Autodesk Inventor part; units mm, degrees
ref_plane "YZ Plane" through (0, 0, 0) normal (1, 0, 0) x (0, 1, 0)
ref_plane "XZ Plane" through (0, 0, 0) normal (0, 1, 0) x (-1, 0, 0)
ref_plane "XY Plane" through (0, 0, 0) normal (0, 0, 1) x (1, 0, 0)
sketch "Sketch1" plane through (0, 0, 0) normal (0, 1, 0) x (-1, 0, 0)
  line L0 (0, 0) -> (-12.7, 0)
  line L1 (-12.7, 0) -> (-12.7, -1.5875)
  line L2 (-12.7, -1.5875) -> (0, -1.5875)
  line L3 (0, -1.5875) -> (0, 0)
  line L4 (0, 0) -> (-4.318, 0)
  line L5 (-4.318, 0) -> (-4.318, -12.7)
  line L6 (-4.318, -12.7) -> (0, -12.7)
  line L7 (0, -12.7) -> (0, 0)
  dimension "d0" = 4.318
  dimension "d1" = 12.7
  dimension "d2" = 12.7
  dimension "d33" = 1.5875
extrude "Extrusion1" add sketch "Sketch1" along normal blind 50.8
sketch "Sketch2" plane through (0, 50.8, 0) normal (0, 1, 0) x (1, 0, 0)
  line L0 (12.7, 0) -> (12.7, 1.5875)
  line L1 (12.7, 1.5875) -> (-4.064, 1.5875)
  line L2 (-4.064, 1.5875) -> (-4.064, -8.5725)
  line L3 (-4.064, -8.5725) -> (12.7, -8.5725)
  line L4 (12.7, -8.5725) -> (12.7, 1.5875)
  line L5 (4.318, 12.7) -> (-4.064, 12.7)
  line L6 (-4.064, 12.7) -> (-4.064, -8.5725)
  line L7 (-4.064, -8.5725) -> (4.318, -8.5725)
  line L8 (4.318, -8.5725) -> (4.318, 12.7)
  dimension "d26" = 10.16
  dimension "d28" = 16.764
extrude "Extrusion2" add sketch "Sketch2" along normal blind 6.35
sketch "Sketch5" plane through (0, 50.8, 0) normal (0, -1, 0) x (1, 0, 0)
  line L0 (12.7, 8.5725) -> (12.7, 0)
  line L1 (-4.064, -12.7) -> (-4.064, 8.5725)
  line L2 (12.7, 8.5725) -> (-4.064, 8.5725)
  line L3 (-4.064, 8.5725) -> (-4.064, 2.1082)
  line L4 (-4.064, 2.1082) -> (12.7, 2.1082)
  line L5 (12.7, 2.1082) -> (12.7, 8.5725)
  line L6 (0, -12.7) -> (-4.064, -12.7)
  line L7 (-4.064, 8.5725) -> (-2.0955, 8.5725)
  line L8 (-2.0955, 8.5725) -> (-2.0955, -12.7)
  line L9 (-2.0955, -12.7) -> (-4.064, -12.7)
  line L10 (-4.064, -12.7) -> (-4.064, 8.5725)
  line L11 (0, -12.7) -> (0, 0)
  line L12 (0, 0) -> (12.7, 0)
  dimension "d29" = 2.0955
  dimension "d30" = 2.1082
extrude "Extrusion4" add sketch "Sketch5" along normal blind 12.7 contours L0 L4 L8 L2 | L8 L4 L1 L2 | L8 L6 L1 L4
sketch "Sketch6" plane through (0, 57.15, 0) normal (0, 1, 0) x (1, 0, 0)
  line L0 (12.7, -8.5725) -> (-4.064, -8.5725)
  line L1 (12.7, -8.5725) -> (-4.064, -8.5725)
  line L2 (-4.064, -8.5725) -> (-4.064, 12.7)
  line L3 (-4.064, 12.7) -> (12.7, 12.7)
  line L4 (12.7, 12.7) -> (12.7, -8.5725)
  point P0 (0, 0)
mirror "Mirror1" about plane through (12.7, 0, 0) normal (1, 0, 0) of "Extrusion4", "Extrusion2", "Extrusion1"
extrude "Extrusion5" cut sketch "Sketch6" against normal blind 254
sketch "Sketch9" plane through (29.464, 38.1, 8.5725) normal (1, 0, 0) x (0, 0, -1)
  line L0 (10.16, 19.05) -> (10.16, -38.1)
  line L1 (21.2725, -38.1) -> (21.2725, 19.05)
  line L2 (21.2725, 19.05) -> (0, 19.05)
  line L3 (21.2725, 0) -> (6.4643, 0)
  line L4 (21.2725, 12.7) -> (8.5725, 12.7)
  point P0 (8.5725, -38.1)
  point P1 (15.7162, 6.35)
  dimension "d62" = 11.1125
  dimension "d64" = 5.5563
  dimension "d72" = 12.7
  dimension "d73" = 6.35
hole "Hole3" at (29.464, 44.45, -7.1437) direction (-1, 0, 0) diameter 5.1562 depth 1.5875 tip angle 118
sketch "Sketch10" plane through (29.464, 38.1, 8.5725) normal (1, 0, 0) x (0, 0, -1)
  circle A0 centre (15.7163, 6.35) radius 2.5781
  line L0 (0, 19.05) -> (0, 0)
  line L1 (0, 0) -> (21.2725, 0)
  line L2 (21.2725, 0) -> (21.2725, 19.05)
  line L3 (21.2725, 19.05) -> (0, 19.05)
  point P0 (8.5725, -38.1)
extrude "Extrusion6" add sketch "Sketch10" along normal blind 2.413
sketch "Sketch11" plane through (27.4955, 38.1, 2.1082) normal (-1, 0, 0) x (0, 0, 1)
  circle A0 centre (-9.252, 6.35) radius 2.5781
  line L0 (6.4643, 0) -> (-14.8082, 0)
  line L1 (-11.8301, 6.35) -> (-6.6739, 6.35)
  line L2 (-6.6739, 6.35) -> (-6.6739, 0)
  line L3 (-6.6739, 0) -> (-11.83, 0)
  line L4 (-11.83, 0) -> (-11.8301, 6.35)
  point P0 (-2.1082, -38.1)
  dimension "d76" = 5.1562
extrude "Extrusion7" cut sketch "Sketch11" against normal blind 1.5875
properties part number "8GrootTelescope"
Check sheet for the modelled part. Datum: model origin and axes. Units: mm. A direction names the side the tool comes from. Give positions to 0.01 mm unless a question says otherwise; leave off trailing zeros. Order: outer loops, then holes, each group sorted by start corner. A loop starts at its lowest first (then second) coordinate and runs counter-clockwise, first axis right, second up. Notation, with made-up numbers: M -4.5,28 L 42.5,28 A24 cw 42.5,50 Z; hole C 49,60 d11. An arc over 180 degrees is marked long. Answer as CSV lines item,"result". Start each with the question number.
Item 1: Cross-section at A-A on y = 49. Enter the section's corners in (x, z), plus the area to 3 significant figures.
Item 2: Mould release check, pull along Z, two halves, no side actions. Record for faces 1 (the face through (22, 0, -5)), 2 (the face through (28, 41, -4.566)), 3 (the face through (22, 48, 8.572)), 4 (the face through (26, 50.8, -3)): +Z half, -Z half, draft (parallel to the pull), parting line (faces both ways), or undercut.
Item 3: Cross-section at B-B on x = 30.75. Enter the section's corners in (y, z), plus the area to 3 significant figures.
Item 4: Cross-section at C-C on x = 18. Enter the section's corners in (y, z), plus the area to 3 significant figures.
Item 5: Gauge pin test, flat ends, axial feed: P1, Ø1.3, axis at y = 44, z = -5.5, coming from the -X side; P2, Ø0.8, axis at y = 45, z = -8, coming from the +X side; P3, Ø2.5, axis at x = 18.5, y = 42, coming from the -Z side. Record the tip position at first contact, or that the pin passes through.
Item 6: Thickness scan on line 1 (Z direction, x = 24.25, y = 50); line 2 (Z direction, x = 30.25, y = 44.45); line 3 (Y direction, x = 30, z = 7). Record the ranges inside material, lowest first. Write a range as [from, to].
Item 7: Cross-section at D-D on y = 12. Enter the section's corners in (x, z), plus the area to 3 significant figures.
Item 8: Tool access check on faces 5 (the face through (20, 45, 2.108)), 6 (the face through (24, 38.1, 3)), 7 (the face through (29.083, 41, -7)), 8 (the face through (21.082, 28, -7)). Record the directions out of +Z, -Z, +X, -X, +Y, -Y that give a thin tool (end or side, any length) a straight path to the whole face; none if there is none.
Established:
1,outline,"M 12.7,-1.59 L 21.08,-1.59 L 21.08,-12.7 L 25.4,-12.7 L 25.4,0 L 12.7,0 Z; M 12.7,2.11 L 27.5,2.11 L 27.5,-12.7 L 31.88,-12.7 L 31.88,8.57 L 12.7,8.57 Z"
1,area,"257 mm^2"
2,face 1,"draft"
2,face 2,"undercut"
2,face 3,"+Z half"
2,face 4,"undercut"
3,outline,"M 38.1,-12.7 L 57.15,-12.7 L 57.15,8.57 L 38.1,8.57 Z; hole C 44.45,-7.14 d5.16"
3,area,"384 mm^2"
4,outline,"M 0,-1.59 L 57.15,-1.59 L 57.15,8.57 L 38.1,8.57 L 38.1,2.11 L 50.8,2.11 L 50.8,0 L 0,0 Z"
4,area,"227 mm^2"
5,P1,"stops at x = 21.08"
5,P2,"stops at x = 25.4"
5,P3,"stops at z = -1.59"
6,line 1,"z = [-12.7, 0], [2.11, 8.57]"
6,line 2,"z = [-12.7, -9.72], [-4.57, 8.57]"
6,line 3,"y = [38.1, 57.15]"
7,outline,"M 12.7,-1.59 L 21.08,-1.59 L 21.08,-12.7 L 25.4,-12.7 L 25.4,0 L 12.7,0 Z"
7,area,"68.1 mm^2"
8,face 5,"-X, -Y"
8,face 6,"+Z, +X, -Y"
8,face 7,"-Y"
8,face 8,"-Z, -X, +Y, -Y"
